Here's how the part is built. I have some questions about the finished solid (model axes, mm). Coordinates: 2 decimals unless noted, no trailing zeros. Write each loop counter-clockwise with the first axis right and the second up, starting at its lowest first coordinate (ties: lowest second). Pieces come first, ordered by that corner, then holes. Notation, with made-up numbers: (5, -25) -> (45, -25) arc R17 ccw to (45, -1) -> close; hole circle Ø6 at (56, -35). An arc over 180 degrees is marked (long way). Put each result on its own line as item: value.
```python
from build123d import *

# Parameters (mm, degrees)
SKETCH1_W          = 160
SKETCH1_H          = 100
BASE_DEPTH         = 10
SKETCH2_R          = 9
ACTUATOR_CUT_DEPTH = 40
CUT_EXTRUDE1_REACH = 12
CUT_EXTRUDE2_REACH = 12
SKETCH5_R          = 3
SKETCH6_R          = 4
CUT_EXTRUDE3_DEPTH = 11


with BuildPart() as part:
    # Sketch1 → base (new body)
    with BuildSketch(Plane(origin=(0, 0, 0), x_dir=(1, 0, 0), z_dir=(0, 1, 0))):
        Rectangle(SKETCH1_W, SKETCH1_H)
    extrude(amount=BASE_DEPTH)

    # Sketch2 → actuator cut (cut)
    with BuildSketch(Plane(origin=(0, 10, 0), x_dir=(1, 0, 0), z_dir=(0, 1, 0))):
        Circle(SKETCH2_R)
    extrude(amount=-ACTUATOR_CUT_DEPTH, mode=Mode.SUBTRACT)

    # Sketch3 → Cut-Extrude1 (cut, up to next)
    with BuildSketch(Plane(origin=(0, 10, 0), x_dir=(1, 0, 0), z_dir=(0, 1, 0)), mode=Mode.PRIVATE) as cut_extrude1_sk1:
        with BuildLine():
            Line((-21.474873734, -16.525126266), (-15.474873734, -10.525126266))
            ThreePointArc((-15.474873734, -10.525126266), (-10.525126266, -10.525126266), (-10.525126266, -15.474873734))
            Line((-10.525126266, -15.474873734), (-16.525126266, -21.474873734))
            ThreePointArc((-16.525126266, -21.474873734), (-21.474873734, -21.474873734), (-21.474873734, -16.525126266))
        make_face()
    cut_extrude1_tool1 = extrude(cut_extrude1_sk1.sketch, amount=-CUT_EXTRUDE1_REACH, mode=Mode.PRIVATE) & part.part
    add(cut_extrude1_tool1.solids().sort_by_distance((-16, 10, 16))[0], mode=Mode.SUBTRACT)
    # Sketch3 → Cut-Extrude1 (cut, up to next)
    with BuildSketch(Plane(origin=(0, 10, 0), x_dir=(1, 0, 0), z_dir=(0, 1, 0)), mode=Mode.PRIVATE) as cut_extrude1_sk2:
        with BuildLine():
            Line((21.474873734, -16.525126266), (15.474873734, -10.525126266))
            ThreePointArc((15.474873734, -10.525126266), (10.525126266, -10.525126266), (10.525126266, -15.474873734))
            Line((10.525126266, -15.474873734), (16.525126266, -21.474873734))
            ThreePointArc((16.525126266, -21.474873734), (21.474873734, -21.474873734), (21.474873734, -16.525126266))
        make_face()
    cut_extrude1_tool2 = extrude(cut_extrude1_sk2.sketch, amount=-CUT_EXTRUDE1_REACH, mode=Mode.PRIVATE) & part.part
    add(cut_extrude1_tool2.solids().sort_by_distance((16, 10, 16))[0], mode=Mode.SUBTRACT)
    # Sketch3 → Cut-Extrude1 (cut, up to next)
    with BuildSketch(Plane(origin=(0, 10, 0), x_dir=(1, 0, 0), z_dir=(0, 1, 0)), mode=Mode.PRIVATE) as cut_extrude1_sk3:
        with BuildLine():
            Line((21.474873734, 16.525126266), (15.474873734, 10.525126266))
            ThreePointArc((15.474873734, 10.525126266), (10.525126266, 10.525126266), (10.525126266, 15.474873734))
            Line((10.525126266, 15.474873734), (16.525126266, 21.474873734))
            ThreePointArc((16.525126266, 21.474873734), (21.474873734, 21.474873734), (21.474873734, 16.525126266))
        make_face()
    cut_extrude1_tool3 = extrude(cut_extrude1_sk3.sketch, amount=-CUT_EXTRUDE1_REACH, mode=Mode.PRIVATE) & part.part
    add(cut_extrude1_tool3.solids().sort_by_distance((16, 10, -16))[0], mode=Mode.SUBTRACT)
    # Sketch3 → Cut-Extrude1 (cut, up to next)
    with BuildSketch(Plane(origin=(0, 10, 0), x_dir=(1, 0, 0), z_dir=(0, 1, 0)), mode=Mode.PRIVATE) as cut_extrude1_sk4:
        with BuildLine():
            Line((-21.474873734, 16.525126266), (-15.474873734, 10.525126266))
            ThreePointArc((-15.474873734, 10.525126266), (-10.525126266, 10.525126266), (-10.525126266, 15.474873734))
            Line((-10.525126266, 15.474873734), (-16.525126266, 21.474873734))
            ThreePointArc((-16.525126266, 21.474873734), (-21.474873734, 21.474873734), (-21.474873734, 16.525126266))
        make_face()
    cut_extrude1_tool4 = extrude(cut_extrude1_sk4.sketch, amount=-CUT_EXTRUDE1_REACH, mode=Mode.PRIVATE) & part.part
    add(cut_extrude1_tool4.solids().sort_by_distance((-16, 10, -16))[0], mode=Mode.SUBTRACT)

    # Sketch5 → Cut-Extrude2 (cut, up to next)
    with BuildSketch(Plane(origin=(0, 10, 0), x_dir=(1, 0, 0), z_dir=(0, 1, 0)), mode=Mode.PRIVATE) as cut_extrude2_sk1:
        with Locations((-40, -40)):
            Circle(SKETCH5_R)
    cut_extrude2_tool1 = extrude(cut_extrude2_sk1.sketch, amount=-CUT_EXTRUDE2_REACH, mode=Mode.PRIVATE) & part.part
    add(cut_extrude2_tool1.solids().sort_by_distance((-40, 10, 40))[0], mode=Mode.SUBTRACT)
    # Sketch5 → Cut-Extrude2 (cut, up to next)
    with BuildSketch(Plane(origin=(0, 10, 0), x_dir=(1, 0, 0), z_dir=(0, 1, 0)), mode=Mode.PRIVATE) as cut_extrude2_sk2:
        with Locations((-40, 40)):
            Circle(SKETCH5_R)
    cut_extrude2_tool2 = extrude(cut_extrude2_sk2.sketch, amount=-CUT_EXTRUDE2_REACH, mode=Mode.PRIVATE) & part.part
    add(cut_extrude2_tool2.solids().sort_by_distance((-40, 10, -40))[0], mode=Mode.SUBTRACT)
    # Sketch5 → Cut-Extrude2 (cut, up to next)
    with BuildSketch(Plane(origin=(0, 10, 0), x_dir=(1, 0, 0), z_dir=(0, 1, 0)), mode=Mode.PRIVATE) as cut_extrude2_sk3:
        with Locations((40, -40)):
            Circle(SKETCH5_R)
    cut_extrude2_tool3 = extrude(cut_extrude2_sk3.sketch, amount=-CUT_EXTRUDE2_REACH, mode=Mode.PRIVATE) & part.part
    add(cut_extrude2_tool3.solids().sort_by_distance((40, 10, 40))[0], mode=Mode.SUBTRACT)
    # Sketch5 → Cut-Extrude2 (cut, up to next)
    with BuildSketch(Plane(origin=(0, 10, 0), x_dir=(1, 0, 0), z_dir=(0, 1, 0)), mode=Mode.PRIVATE) as cut_extrude2_sk4:
        with Locations((40, 40)):
            Circle(SKETCH5_R)
    cut_extrude2_tool4 = extrude(cut_extrude2_sk4.sketch, amount=-CUT_EXTRUDE2_REACH, mode=Mode.PRIVATE) & part.part
    add(cut_extrude2_tool4.solids().sort_by_distance((40, 10, -40))[0], mode=Mode.SUBTRACT)

    # Sketch6 → Cut-Extrude3 (cut, through all)
    with BuildSketch(Plane.XZ):
        with Locations((-40, 40)):
            Circle(SKETCH6_R)
        with Locations((40, 40)):
            Circle(SKETCH6_R)
        with Locations((40, -40)):
            Circle(SKETCH6_R)
        with Locations((-40, -40)):
            Circle(SKETCH6_R)
    extrude(amount=-CUT_EXTRUDE3_DEPTH, mode=Mode.SUBTRACT)


solid = part.part
```
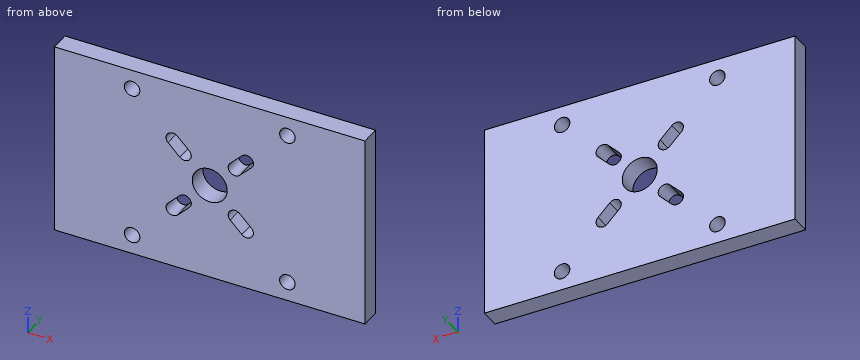
Item 1: Please list where these lines run through material, in increasing order: line 1 along Z through (x, y) = (40, 7.75); line 2 along X through (y, z) = (7.25, -16.5); line 3 along Z through (x, y) = (-43, 6). Write a range as from..to.
Output:
line 1: z = -50..-44, -36..36, 44..50
line 2: x = -80..-21.45, -11.55..11.55, 21.45..80
line 3: z = -50..-42.65, -37.35..37.35, 42.65..50
Item 2: Imagine slicing it at D-D on z = -19. Write out the boundary of the cut face in (x, y), then the cut area to 3 significant figures.
Output:
outline: (-80, 0) -> (-22.5, 0) -> (-22.5, 10) -> (-80, 10) -> close; (-14.05, 0) -> (14.05, 0) -> (14.05, 10) -> (-14.05, 10) -> close; (22.5, 0) -> (80, 0) -> (80, 10) -> (22.5, 10) -> close
area: 1,430 mm²
Item 3: Imagine slicing it at C-C on y = 7.25. State how many separate pieces and enclosed holes the cut face has, then the cut area to 3 significant figures.
Output:
separate pieces: 1
enclosed holes: 9
area: 15,200 mm²
Item 4: Imagine slicing it at B-B on x = -40. Write out the boundary of the cut face in (y, z).
Output:
outline: (0, -50) -> (10, -50) -> (10, -44) -> (0, -44) -> close; (0, -36) -> (10, -36) -> (10, 36) -> (0, 36) -> close; (0, 44) -> (10, 44) -> (10, 50) -> (0, 50) -> close
Item 5: Imagine slicing it at A-A on x = 0. Write out the boundary of the cut face in (y, z).
Output:
outline: (0, -50) -> (10, -50) -> (10, -9) -> (0, -9) -> close; (0, 9) -> (10, 9) -> (10, 50) -> (0, 50) -> close
